Input: part model. Units: mm. Frame: model coordinates. Face numbers are marked on the shaded views. A direction names the side the tool comes from. Give positions to 0.01 mm unless a question says otherwise; leave off trailing zeros. Loops run counter-clockwise (first coordinate to the right, second up) from the corner with the lowest first, then second, coordinate; pieces in that order, holes last. Notation, with made-up numbers: (45.5, 49.5) -> (63.5, 49.5) arc R21 cw to (63.5, 60.5) -> close; hole circle Ø10 at (56.5, 34). An arc over 180 degrees is marked (long way). Use CSV: the item, a comma, the result in double quotes.
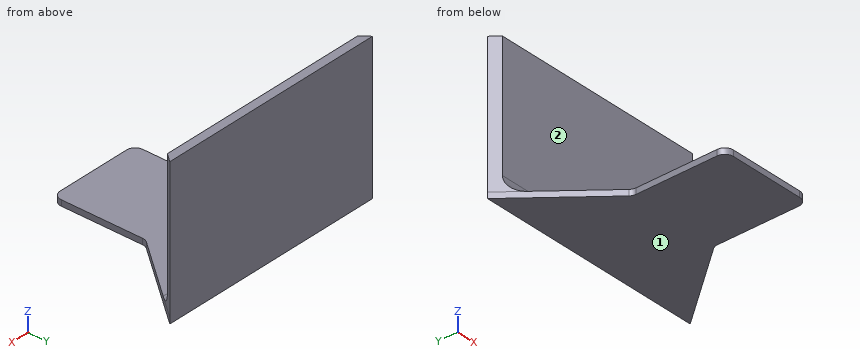
```python
from build123d import *

# Parameters (mm, degrees)
SIDE_EXTRUDE_DEPTH         = 2
TOP_EXTRUDE_DEPTH          = 48
FILLET_BETWEEN_SIDES_5MM_R = 5


with BuildPart() as part:
    # Sketch1 → Side extrude (new body)
    with BuildSketch(Plane.XY.offset(55.601550083)):
        with BuildLine():
            Line((93.845211173, 26.628512047), (21.944630571, 26.628512047))
            Line((21.944630571, 26.628512047), (18.071324489, 26.628512047))
            Line((18.071324489, 26.628512047), (41.218517255, -1.714989299))
            ThreePointArc((41.218517255, -1.714989299), (41.720764918, -2.60531677), (41.894920872, -3.612593011))
            Line((41.894920872, -3.612593011), (41.894920872, -31.543238626))
            ThreePointArc((41.894920872, -31.543238626), (42.773600528, -33.66455897), (44.894920872, -34.543238626))
            Line((44.894920872, -34.543238626), (70.894920872, -34.543238626))
            ThreePointArc((70.894920872, -34.543238626), (73.016241216, -33.66455897), (73.894920872, -31.543238626))
            Line((73.894920872, -31.543238626), (73.894920872, -3.612593011))
            ThreePointArc((73.894920872, -3.612593011), (74.069076826, -2.60531677), (74.571324489, -1.714989299))
            Line((74.571324489, -1.714989299), (97.718517255, 26.628512047))
            Line((97.718517255, 26.628512047), (93.845211173, 26.628512047))
        make_face()
    extrude(amount=SIDE_EXTRUDE_DEPTH)

    # Sketch2 → Top extrude (add)
    with BuildSketch(Plane.XY.offset(57.601550083)):
        Polygon((97.718517255, 26.628512047), (18.071324489, 26.628512047), (20.521324489, 23.628512047), (95.268517255, 23.628512047), align=None)
    extrude(amount=TOP_EXTRUDE_DEPTH)

    # Fillet between sides 5mm
    fillet_between_sides_5mm_edges = [part.edges().sort_by_distance(p)[0] for p in [
        (57.894920872, 23.628512047, 57.601550083),
    ]]
    fillet(fillet_between_sides_5mm_edges, radius=FILLET_BETWEEN_SIDES_5MM_R)


solid = part.part
```
1) Contact query for flat-ended pins moving along their axis: pin 1 (1 mm diameter, centred on y = -12.5, z = 56.5, fed in from -X); pin 2 (4 mm diameter, centred on x = 38.5, y = 1, fed in from +Z); pin 3 (1 mm diameter, centred on y = -14, z = 56, fed in from +X). Output: stop coordinate, or through.
From the geometry:
pin 1,"stops at x = 41.89"
pin 2,"stops at z = 57.6"
pin 3,"stops at x = 73.89"
2) Section query B-B (y = -21.5). Return loops of the section in (x, z), then the cut area to 3 significant figures.
From the geometry:
outline,"(41.89, 55.6) -> (73.89, 55.6) -> (73.89, 57.6) -> (41.89, 57.6) -> close"
area,"64.0 mm^2"
3) Section query D-D (x = 38). Return loops of the section in (y, z), then the cut area to 3 significant figures.
From the geometry:
outline,"(2.23, 55.6) -> (26.63, 55.6) -> (26.63, 105.6) -> (23.63, 105.6) -> (23.63, 62.6) arc R5 cw to (18.63, 57.6) -> (2.23, 57.6) -> close"
area,"198 mm^2"
4) Section query A-A (x = 62.5). Return loops of the section in (y, z), then the cut area to 3 significant figures.
From the geometry:
outline,"(-34.54, 55.6) -> (26.63, 55.6) -> (26.63, 105.6) -> (23.63, 105.6) -> (23.63, 62.6) arc R5 cw to (18.63, 57.6) -> (-34.54, 57.6) -> close"
area,"272 mm^2"
5) Reachability of the marked faces 1 and 2 from +Z, -Z, +X, -X, +Y, -Y: full face, straight path, thin tool, end or side. Return the list, or none.
From the geometry:
face 1,"-Z, +X, -X, +Y, -Y"
face 2,"+Z, +X, -X, -Y"
6) Section query C-C (z = 83.5). Return loops of the section in (x, y), then the cut area to 3 significant figures.
From the geometry:
outline,"(18.07, 26.63) -> (20.52, 23.63) -> (95.27, 23.63) -> (97.72, 26.63) -> close"
area,"232 mm^2"
7) Ray query, line 1 (Y direction, x = 40.5, z = 90); line 2 (Z direction, x = 69, y = 1.5); line 3 (Z direction, x = 67, y = 20). Return the intervals inside material, ascending.
From the geometry:
line 1,"y = 23.63 to 26.63"
line 2,"z = 55.6 to 57.6"
line 3,"z = 55.6 to 57.79"
